from build123d import *

# Parameters (mm, degrees)
EXTRUDE_1_DEPTH     = 8
CUT_EXTRUDE_1_DEPTH = 8.5
EXTRUDE_2_DEPTH     = 8
EXTRUDE_3_DEPTH     = 10
SKETCH_7_R          = 5.5
CUT_EXTRUDE_2_DEPTH = 22
EXTRUDE_5_DEPTH     = 26
CUT_EXTRUDE_4_DEPTH = 21
CHAMFER_6_SIZE      = 5
CHAMFER_8_SIZE      = 10
SKETCH_13_W         = 210
SKETCH_13_H         = 10
CUT_EXTRUDE_5_DEPTH = 15
SKETCH_14_W         = 160
SKETCH_14_H         = 5
CUT_EXTRUDE_6_DEPTH = 10
SKETCH_16_R         = 2
CUT_EXTRUDE_7_DEPTH = 10
SKETCH_18_W         = 109.386418102
SKETCH_18_H         = 16
EXTRUDE_7_DEPTH     = 2
CHAMFER_10_SIZE     = 2


with BuildPart() as part:
    # 草图1 → 凸台-拉伸1 (new body)
    with BuildSketch(Plane.XY):
        Polygon((-60, 0), (60, 0), (115, 270), (-115, 270), align=None)
    extrude(amount=EXTRUDE_1_DEPTH)

    # 草图2 → 切除-拉伸1 (cut)
    with BuildSketch(Plane.XY.offset(8)):
        with BuildLine():
            Line((0.005000474, 0.310000947), (0, 0.3))
            Line((0, 0.3), (17.48870838, 0.3))
            Line((17.48870838, 0.3), (12.108893566, 26.71))
            Line((12.108893566, 26.71), (0, 26.71))
            ThreePointArc((0, 26.71), (-13.199999763, 13.507499763), (0.005000474, 0.310000947))
        make_face()
    extrude(amount=-CUT_EXTRUDE_1_DEPTH, mode=Mode.SUBTRACT)

    # 草图5 → 凸台-拉伸2 (add)
    with BuildSketch(Plane(origin=(0, 0, 0), x_dir=(-1, 0, 0), z_dir=(0, 0, -1))):
        Polygon((60, 0), (115, 270), (-115, 270), (-60, 0), align=None)
    extrude(amount=EXTRUDE_2_DEPTH)

    # 草图6 → 凸台-拉伸3 (add)
    with BuildSketch(Plane.XY.offset(8)):
        Polygon((-115, 270), (-60, 0), (60, 0), (115, 270), align=None)
    extrude(amount=EXTRUDE_3_DEPTH)

    # 草图7 → 切除-拉伸2 (cut)
    with BuildSketch(Plane.XY.offset(18)):
        with Locations((0, 13.51)):
            Circle(SKETCH_7_R)
    extrude(amount=-CUT_EXTRUDE_2_DEPTH, mode=Mode.SUBTRACT)

    # 草图9 → 凸台-拉伸5 (add)
    with BuildSketch(Plane.XY.offset(18)):
        Polygon((-57.962962963, -10), (-60, 0), (60, 0), (57.962962963, -10), align=None)
    extrude(amount=-EXTRUDE_5_DEPTH)

    # 草图12 → 切除-拉伸4 (cut)
    with BuildSketch(Plane.XY.offset(-8)):
        Polygon((54.693209051, 0), (-54.693209051, 0), (-52.656172014, -10), (52.656172014, -10), align=None)
    extrude(amount=CUT_EXTRUDE_4_DEPTH, mode=Mode.SUBTRACT)

    # 倒角6
    chamfer_6_edges = [part.edges().sort_by_distance(p)[0] for p in [
        (0, 0, -8),
    ]]
    chamfer(chamfer_6_edges, length=CHAMFER_6_SIZE)

    # 倒角8
    chamfer_8_edges = [part.edges().sort_by_distance(p)[0] for p in [
        (55.309567488, -10, -8),
        (-55.309567488, -10, -8),
    ]]
    chamfer(chamfer_8_edges, length=CHAMFER_8_SIZE)

    # 草图13 → 切除-拉伸5 (cut)
    with BuildSketch(Plane(origin=(0, 270, 0), x_dir=(1, 0, 0), z_dir=(0, 1, 0))):
        with Locations((0, -5)):
            Rectangle(SKETCH_13_W, SKETCH_13_H)
    extrude(amount=-CUT_EXTRUDE_5_DEPTH, mode=Mode.SUBTRACT)

    # 草图14 → 切除-拉伸6 (cut)
    with BuildSketch(Plane.XY.offset(18)):
        with Locations((0, 173.51)):
            Rectangle(SKETCH_14_W, SKETCH_14_H)
    extrude(amount=-CUT_EXTRUDE_6_DEPTH, mode=Mode.SUBTRACT)

    # 草图16 → 切除-拉伸7 (cut)
    with BuildSketch(Plane.XY.offset(18)):
        with Locations((-77.25, 256.1425573)):
            Circle(SKETCH_16_R)
        with Locations((-90, 237)):
            Circle(SKETCH_16_R)
        with Locations((-64.5, 237)):
            Circle(SKETCH_16_R)
        with Locations((77.25, 256.1425573)):
            Circle(SKETCH_16_R)
        with Locations((64.5, 237)):
            Circle(SKETCH_16_R)
        with Locations((90, 237)):
            Circle(SKETCH_16_R)
        with Locations((-55, 154.6525573)):
            Circle(SKETCH_16_R)
        with Locations((-42.25, 135.51)):
            Circle(SKETCH_16_R)
        with Locations((55, 154.6525573)):
            Circle(SKETCH_16_R)
        with Locations((42.25, 135.51)):
            Circle(SKETCH_16_R)
        with Locations((67.75, 135.51)):
            Circle(SKETCH_16_R)
        with Locations((-67.75, 135.51)):
            Circle(SKETCH_16_R)
    extrude(amount=-CUT_EXTRUDE_7_DEPTH, mode=Mode.SUBTRACT)

    # 草图18 → 凸台-拉伸7 (add)
    with BuildSketch(Plane.XZ):
        with Locations((0, 5)):
            Rectangle(SKETCH_18_W, SKETCH_18_H)
    extrude(amount=EXTRUDE_7_DEPTH)

    # 倒角10
    chamfer_10_edges = [part.edges().sort_by_distance(p)[0] for p in [
        (0, -2, -3),
    ]]
    chamfer(chamfer_10_edges, length=CHAMFER_10_SIZE - 0.0001)  # a hair under: the kernel refuses the full size


solid = part.part
The listing builds one solid part. Answer for the finished solid, in the listing's coordinates (mm). A direction names the side the tool comes from. Give positions to 0.01 mm unless a question says otherwise; leave off trailing zeros. Loops run counter-clockwise (first coordinate to the right, second up) from the corner with the lowest first, then second, coordinate; pieces in that order, holes last. Notation, with made-up numbers: (10.25, -19) - (69.25, -19) arc R23 ccw to (69.25, 13) - close; hole circle Ø7 at (-14, -14.5). An arc over 180 degrees is marked (long way). Write each question's results on one line, items separated by ' | '.
1. Find section A-A, the plane y = 121. Write down the section's boundary in (x, z).
Resolved:
outline: (-84.65, -8) - (84.65, -8) - (84.65, 18) - (-84.65, 18) - close
2. Flat-ended cylindrical pins translate along their axes: P1, Ø4, axis at y = 195.5, z = 4.5, coming from the +X side; P2, Ø12, axis at y = 219, z = 12, coming from the -X side; P3, Ø6, axis at x = -47, z = 0.5, coming from the -Y side. Find the tip coordinate at first contact, or state that the pin passes through.
Resolved:
P1: stops at x = 100.23 | P2: stops at x = -105.83 | P3: stops at y = -2
3. For a pull along X with two mould halves and no side action, classify faces 6 (the face through (0, -10, 14)), 7 (the face through (-1, 176.01, 13)) as +X half, -X half, draft (parallel to the pull), parting line (faces both ways), or undercut.
Resolved:
face 6: draft | face 7: undercut
4. Which of the six approach directions +Z, -Z, +X, -X, +Y, -Y give full straight-line access (tool end or side, diameter ignored) to faces 1 (the face through (-1.19, 8.14, -1.97)), 2 (the face through (-13.197, 13.798, 4.056)), 3 (the face through (-56, -5, -3)), 4 (the face through (53.823, -4.272, 2.353)), 5 (the face through (105, 263, 5))?
Resolved:
face 1: +Z | face 2: none | face 3: -Z, +X, -X, -Y | face 4: -Z | face 5: +Y
5. Find section B-B, the plane y = 165. Write down the section's boundary in (x, z).
Resolved:
outline: (-93.61, -8) - (93.61, -8) - (93.61, 18) - (-93.61, 18) - close
6. Consider probe 1 along Y at (x, z) = (-42.25, 10.5); probe 2 along X at (y, z) = (135.51, 15); probe 3 along X at (y, z) = (237, 11.5). Determine where each line is inside the solid, lowest interval first. Write a range as from..to.
Resolved:
probe 1: y = -2..133.51, 137.51..171.01, 176.01..270 | probe 2: x = -87.6..-69.75, -65.75..-44.25, -40.25..40.25, 44.25..65.75, 69.75..87.6 | probe 3: x = -108.28..-92, -88..-66.5, -62.5..62.5, 66.5..88, 92..108.28
